Geometry: see drawing. Coordinates: mm, zero at the bounding-box minimum. A direction names the side the tool comes from. Coordinates: 2 decimals unless noted, no trailing zeros. Write each loop counter-clockwise with the first axis right and the second up, starting at its lowest first coordinate (ties: lowest second). Pieces come first, ordered by that corner, then holes.
1) Set-up query: the marked faces 5 and 6. Return all of +Z, -Z, +X, -X, +Y, -Y with unobstructed straight access to the full face (end or side cutting, diameter ignored); none if empty.
2) Section query D-D (y = 18.75). Output: boundary loops of the cut face in (x, z), then the cut area to 3 significant figures.
3) Section query A-A (x = 6.5). Output: boundary loops of the cut face in (y, z).
4) Pin query (flat end, axial travel): pin 1 Ø1 at (x, z) = (5, 0.5) entering from -Y. Return the tip coordinate at first contact, or that it passes through.
5) Section query C-C (z = 0.6). Output: boundary loops of the cut face in (x, y), then the cut area to 3 significant figures.
6) Line query: L1, parallel to X at y = 22, z = 1.75; L2, parallel to Y at x = 4, z = 1.75; L3, parallel to Y at x = 8.25, z = 1. Output: solid intervals per line, ascending.
7) Draft query along X for the marked faces 1, 2, 3 and 4. Return one class per face: pulls with the +X half, pulls with the -X half, needs draft (parallel to the pull), parting line crosses it, or undercut.
8) Section query B-B (y = 6.5). Output: boundary loops of the cut face in (x, z), then the cut area to 3 significant figures.
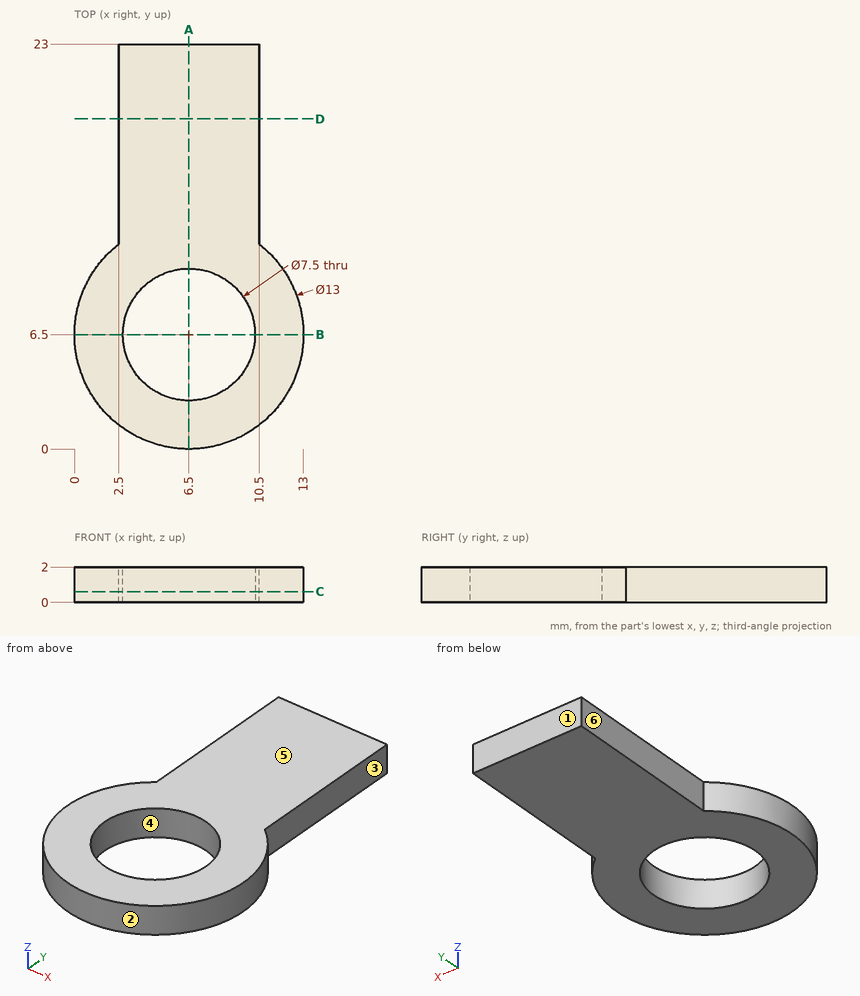
Answer:
1. face 5: +Z, +X, -X, +Y, -Y
1. face 6: +Z, -Z, -X, +Y
2. outline: (2.5, 0) - (10.5, 0) - (10.5, 2) - (2.5, 2) - close
2. area: 16.0 mm2
3. outline: (0, 0) - (2.75, 0) - (2.75, 2) - (0, 2) - close; (10.25, 0) - (23, 0) - (23, 2) - (10.25, 2) - close
4. pin 1: stops at y = 0.08
5. outline: (2.5, 11.62) arc R6.5 ccw (long way) to (10.5, 11.62) - (10.5, 23) - (2.5, 23) - close; hole circle Ø7.5 at (6.5, 6.5)
5. area: 172 mm2
6. L1: x = 2.5 to 10.5
6. L2: y = 0.5 to 3.7, 9.3 to 23
6. L3: y = 0.24 to 3.18, 9.82 to 23
7. face 1: needs draft
7. face 2: parting line crosses it
7. face 3: pulls with the +X half
7. face 4: undercut
8. outline: (0, 0) - (2.75, 0) - (2.75, 2) - (0, 2) - close; (10.25, 0) - (13, 0) - (13, 2) - (10.25, 2) - close
8. area: 11.0 mm2
